```python
from build123d import *

# Parameters (mm, degrees)
BOSS_EXTRUDE1_DEPTH = 44.45
SKETCH2_R           = 3.429
CUT_EXTRUDE1_DEPTH  = 44.45
SKETCH3_R           = 3.429
CUT_EXTRUDE2_DEPTH  = 44.45
CUT_EXTRUDE3_DEPTH  = 5.588
CUT_EXTRUDE4_DEPTH  = 5.588
BOSS_EXTRUDE2_DEPTH = 3.175
FILLET1_R           = 2.54
SKETCH7_R           = 1.5875
BOSS_EXTRUDE3_DEPTH = 5.08


with BuildPart() as part:
    # Sketch1 → Boss-Extrude1 (new body)
    with BuildSketch(Plane.XY):
        Polygon((0, 0), (63.5, 0), (63.5, 10.16), (7.431912016, 10.16), (53.213794099, 42.527418233), (47.348550945, 50.823472882), (-4.50179061, 14.165703165), align=None)
    extrude(amount=BOSS_EXTRUDE1_DEPTH)

    # Sketch2 → Cut-Extrude1 (cut)
    with BuildSketch(Plane(origin=(0, 10.16, 0), x_dir=(1, 0, 0), z_dir=(0, 1, 0))):
        with Locations((53.34, -34.925)):
            Circle(SKETCH2_R)
        with Locations((53.34, -9.525)):
            Circle(SKETCH2_R)
        with Locations((27.94, -9.525)):
            Circle(SKETCH2_R)
        with Locations((27.94, -34.925)):
            Circle(SKETCH2_R)
    extrude(amount=-CUT_EXTRUDE1_DEPTH, mode=Mode.SUBTRACT)

    # Sketch3 → Cut-Extrude2 (cut)
    with BuildSketch(Plane(origin=(-2.312443215, 3.270820114, 0), x_dir=(0, 0, -1), z_dir=(0.577287712, -0.816540812, 0))):
        with Locations((-9.525, 32.44179061)):
            Circle(SKETCH3_R)
        with Locations((-9.525, 57.84179061)):
            Circle(SKETCH3_R)
        with Locations((-34.925, 57.84179061)):
            Circle(SKETCH3_R)
        with Locations((-34.925, 32.44179061)):
            Circle(SKETCH3_R)
    extrude(amount=-CUT_EXTRUDE2_DEPTH, mode=Mode.SUBTRACT)

    # Sketch4 → Cut-Extrude3 (cut)
    with BuildSketch(Plane(origin=(0, 10.16, 0), x_dir=(1, 0, 0), z_dir=(0, 1, 0))):
        Polygon((22.225, -31.625443212), (22.225, -38.224556788), (27.94, -41.524113577), (33.655, -38.224556788), (33.655, -31.625443212), (27.94, -28.325886423), align=None)
        Polygon((47.625, -31.625443212), (47.625, -38.224556788), (53.34, -41.524113577), (59.055, -38.224556788), (59.055, -31.625443212), (53.34, -28.325886423), align=None)
        Polygon((22.225, -6.225443212), (22.225, -12.824556788), (27.94, -16.124113577), (33.655, -12.824556788), (33.655, -6.225443212), (27.94, -2.925886423), align=None)
        Polygon((47.625, -6.225443212), (47.625, -12.824556788), (53.34, -16.124113577), (59.055, -12.824556788), (59.055, -6.225443212), (53.34, -2.925886423), align=None)
    extrude(amount=-CUT_EXTRUDE3_DEPTH, mode=Mode.SUBTRACT)

    # Sketch5 → Cut-Extrude4 (cut)
    with BuildSketch(Plane(origin=(-2.312443215, 3.270820114, 0), x_dir=(0, 0, -1), z_dir=(0.577287712, -0.816540812, 0))):
        Polygon((-2.925886423, 57.84179061), (-6.225443212, 63.55679061), (-12.824556788, 63.55679061), (-16.124113577, 57.84179061), (-12.824556788, 52.12679061), (-6.225443212, 52.12679061), align=None)
        Polygon((-28.325886423, 57.84179061), (-31.625443212, 63.55679061), (-38.224556788, 63.55679061), (-41.524113577, 57.84179061), (-38.224556788, 52.12679061), (-31.625443212, 52.12679061), align=None)
        Polygon((-2.925886423, 32.44179061), (-6.225443212, 38.15679061), (-12.824556788, 38.15679061), (-16.124113577, 32.44179061), (-12.824556788, 26.72679061), (-6.225443212, 26.72679061), align=None)
        Polygon((-28.325886423, 32.44179061), (-31.625443212, 38.15679061), (-38.224556788, 38.15679061), (-41.524113577, 32.44179061), (-38.224556788, 26.72679061), (-31.625443212, 26.72679061), align=None)
    extrude(amount=-CUT_EXTRUDE4_DEPTH, mode=Mode.SUBTRACT)

    # Sketch6 → Boss-Extrude2 (add, symmetric)
    with BuildSketch(Plane.XY.offset(22.225)):
        Polygon((7.431912016, 10.16), (34.372680379, 37.100768363), (45.531912016, 10.16), align=None)
    extrude(amount=BOSS_EXTRUDE2_DEPTH, both=True)

    # Fillet1
    fillet1_edges = [part.edges().sort_by_distance(p)[0] for p in [
        (-4.50179061, 14.165703165, 22.225),
        (47.348550945, 50.823472882, 22.225),
        (53.213794099, 42.527418233, 22.225),
        (7.431912016, 10.16, 34.925),
        (63.5, 10.16, 22.225),
        (63.5, 0, 22.225),
        (0, 0, 22.225),
        (7.431912016, 10.16, 9.525),
        (22.166849982, 20.577481285, 19.05),
        (36.901787948, 30.99496257, 22.225),
        (22.166849982, 20.577481285, 25.4),
        (45.531912016, 10.16, 22.225),
        (26.481912016, 10.16, 25.4),
        (26.481912016, 10.16, 19.05),
    ]]
    fillet(fillet1_edges, radius=FILLET1_R)

    # Sketch7 → Boss-Extrude3 (add)
    with BuildSketch(Plane(origin=(0, 2.54, 0), x_dir=(-1, 0, 0), z_dir=(0, -1, 0))):
        with BuildLine():
            Line((-63.5, 0), (-63.5, -44.45))
            ThreePointArc((-63.5, -44.45), (-72.480256121, -40.730256121), (-76.2, -31.75))
            Line((-76.2, -31.75), (-76.2, -12.7))
            ThreePointArc((-76.2, -12.7), (-72.480256121, -3.719743879), (-63.5, 0))
        make_face()
        with Locations((-69.85, -12.7)):
            Circle(SKETCH7_R, mode=Mode.SUBTRACT)
        with Locations((-69.85, -31.75)):
            Circle(SKETCH7_R, mode=Mode.SUBTRACT)
    extrude(amount=-BOSS_EXTRUDE3_DEPTH)


solid = part.part
```
CAD build for the part. Positions are in the model's coordinates, mm. A direction names the side the tool comes from. Give positions to 0.01 mm unless a question says otherwise; leave off trailing zeros. Order: outer loops, then holes, each group sorted by start corner. A loop starts at its lowest first (then second) coordinate and runs counter-clockwise, first axis right, second up.
(1) Saw through at C-C, the plane x = 4.5. Give the cut face in (y, z), then the cut area to 3 significant figures.
(2) Drill centre lines: L1, parallel to Z at x = 53.34, y = 3.05; L2, parallel to Z at x = 68.5, y = 5; L3, parallel to Y at x = 57, z = 17. Where is each one in solid material? Low to high.
(3) Tool access for faces 1 (the flat face through (41.03, 37.29, 39.9)), 2 (the cylindrical face through (24.514, 2.318, 9.374)), 3 (the cylindrical face through (26.504, 22.757, 26.164)): list every direction of +Z, -Z, +X, -X, +Y, -Y with a clear straight run to the whole face (end or side of a thin tool).
(4) Saw through at D-D, the plane z = 36. State how many separate pieces and enclosed holes the cut face has, then the cut area to 3 significant figures.
(5) Mould opens along X. For faces 4 (the flat face through (33.655, 7, 10)), 5 (the cylindrical face through (72.38, 5.04, 40.83)) say: released by +X, released by -X, zero draft, split by the parting line, or undercut.
(6) Flat gauge pins, fed straight in: pin 1 (4 mm diameter, centred on y = 21.5, z = 39, fed in from +X); pin 2 (3 mm diameter, centred on y = 8, z = 34.5, fed in from +X); pin 3 (4 mm diameter, centred on x = 39, z = 38, fed in from +Y). Where does each tip first touch, or does it go through?
(7) Saw through at A-A, the plane x = 69.85. Give the cut face in (y, z), then the cut area to 3 significant figures.
(8) Saw through at B-B, the plane z = 23. Give the cut face in (x, y) (3 decimals), then the cut area to 3 significant figures.
Results found:
1. outline: (0, 0) - (20.53, 0) - (20.53, 44.45) - (0, 44.45) - close
1. area: 913 mm2
2. L1: z = 0 to 6.1, 12.95 to 31.5, 38.35 to 44.45
2. L2: z = 1.03 to 11.86, 13.54 to 30.91, 32.59 to 43.42
2. L3: y = 0 to 10.16
3. face 1: none
3. face 2: -Y
3. face 3: +Z, +X
4. separate pieces: 5
4. enclosed holes: 0
4. area: 982 mm2
5. face 4: undercut
5. face 5: released by +X
6. pin 1: stops at x = 23.44
6. pin 2: stops at x = 76.13
6. pin 3: stops at y = 46.34
7. outline: (2.54, 1.7) - (7.62, 1.7) - (7.62, 11.11) - (2.54, 11.11) - close; (2.54, 14.29) - (7.62, 14.29) - (7.62, 30.16) - (2.54, 30.16) - close; (2.54, 33.34) - (7.62, 33.34) - (7.62, 42.75) - (2.54, 42.75) - close
7. area: 176 mm2
8. outline: (-3.939, 12.395) - (-0.563, 1.771) arc R2.54 ccw to (1.858, 0) - (60.96, 0) arc R2.54 ccw to (63.5, 2.54) - (76.2, 2.54) - (76.2, 7.62) - (63.5, 7.62) arc R2.54 ccw to (60.96, 10.16) - (47.229, 10.16) arc R2.54 cw to (44.882, 11.728) - (37.678, 29.12) arc R2.54 cw to (38.559, 32.166) - (51.14, 41.061) arc R2.54 ccw to (51.747, 44.601) - (48.815, 48.749) arc R2.54 ccw to (45.275, 49.357) - (-2.985, 15.238) arc R2.54 ccw to start
8. area: 1,750 mm2
